Can you work these out from the drawing? Everything is in mm from the part's minimum corner. Round coordinates to 2 decimals unless told otherwise and drop trailing zeros. Loops run counter-clockwise (first coordinate to the right, second up) from the corner with the lowest first, then second, coordinate; pieces in that order, holes last. Notation, with made-up numbers: (-14.75, -25.5) -> (33.25, -25.5) arc R25 cw to (33.25, -13.5) -> close; hole circle Ø5 at (53, 18.25). An arc over 180 degrees is marked (long way). One line per item, written item: value.
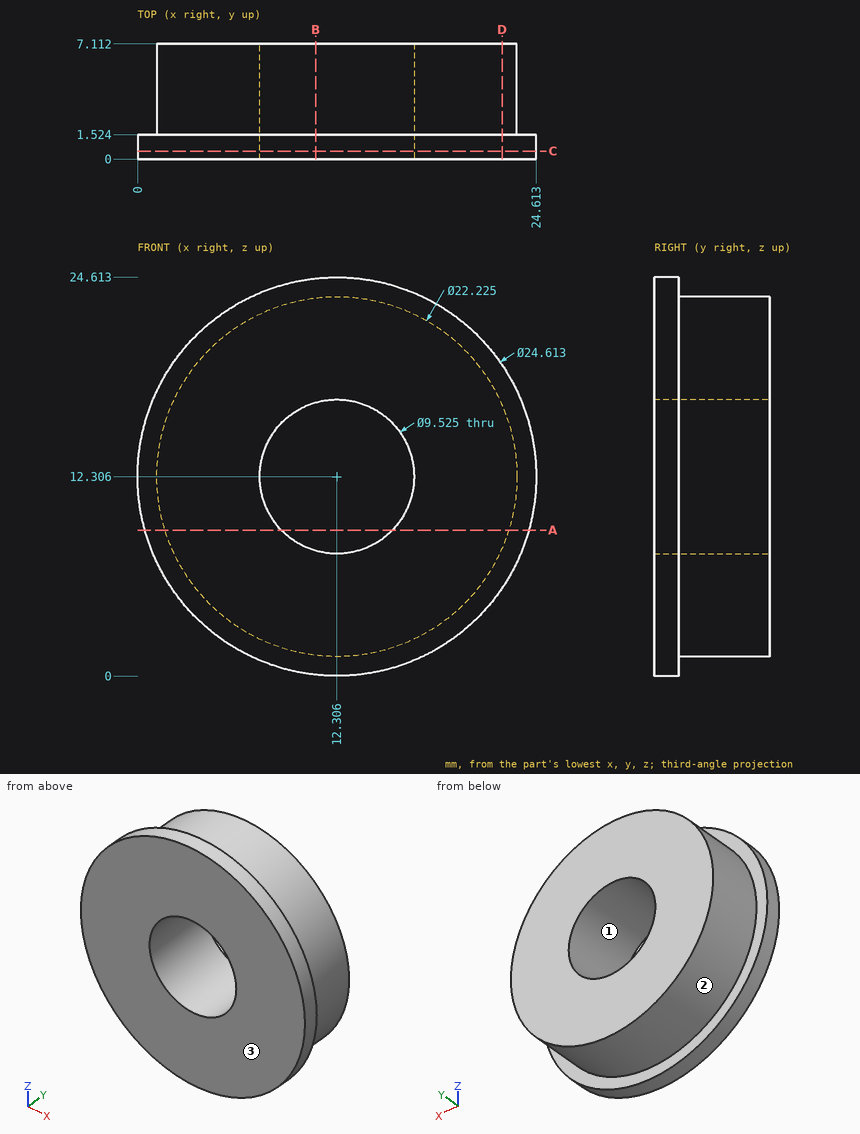
(1) If we section it at D-D, the plane x = 22.5: Please give me the cut outline in (y, z).
Recorded:
outline: (0, 5.41) -> (1.52, 5.41) -> (1.52, 7.88) -> (7.11, 7.88) -> (7.11, 16.73) -> (1.52, 16.73) -> (1.52, 19.2) -> (0, 19.2) -> close
(2) Thinking about a two-plate mould opening in X: for the marked faces 1, 2 and 3, which applies, released by +X, released by -X, zero draft, split by the parting line, or undercut?
Recorded:
face 1: undercut
face 2: split by the parting line
face 3: zero draft
(3) If we section it at A-A, the plane z = 9: Please give me the cut outline in (x, y) (1 decimal), then the cut area to 3 significant figures.
Recorded:
outline: (0.5, 0) -> (8.9, 0) -> (8.9, 7.1) -> (1.7, 7.1) -> (1.7, 1.5) -> (0.5, 1.5) -> close; (15.7, 0) -> (24.2, 0) -> (24.2, 1.5) -> (22.9, 1.5) -> (22.9, 7.1) -> (15.7, 7.1) -> close
area: 106 mm²
(4) If we section it at B-B, the plane x = 11: Please give me the cut outline in (y, z).
Recorded:
outline: (0, 0.07) -> (1.52, 0.07) -> (1.52, 1.27) -> (7.11, 1.27) -> (7.11, 7.73) -> (0, 7.73) -> close; (0, 16.89) -> (7.11, 16.89) -> (7.11, 23.34) -> (1.52, 23.34) -> (1.52, 24.54) -> (0, 24.54) -> close
(5) If I drill on L1, parallel to Z at x = 14.75, y = 3 (1 decimal); L2, parallel to X at y = 0.5, z = 13 (1 decimal); L3, parallel to Z at x = 8.75, y = 3 (1 decimal), over which ranges is the centre line in solid material (lowest first)?
Recorded:
L1: 1.5 to 8.2, 16.4 to 23.1
L2: 0 to 7.6, 17 to 24.6
L3: 1.8 to 9.1, 15.5 to 22.8
(6) I'm going to push a flat-ended pin straight in: pin 1 Ø4 at (y, z) = (1.5, 16) entering from -X. Where does the tip first touch, or does it pass through?
Recorded:
pin 1: x = 0.12
(7) If we section it at C-C, the plane y = 0.5: Please give me the cut outline in (x, z) (1 decimal).
Recorded:
outline: circle Ø24.6 at (12.3, 12.3); hole circle Ø9.5 at (12.3, 12.3)
